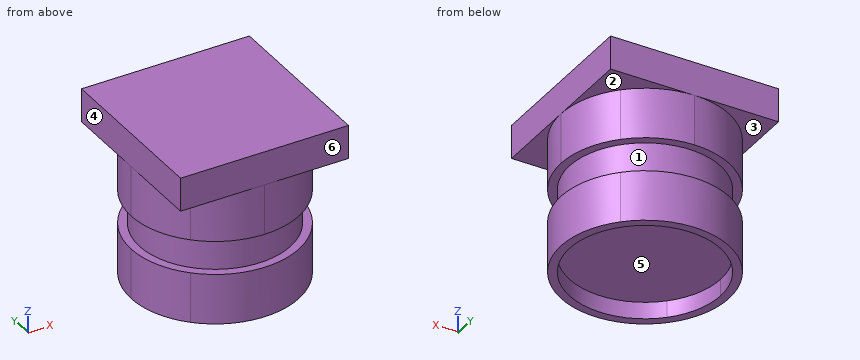
```python
from build123d import *

# Parameters (mm, degrees)
ESQUISSE1_W             = 10
ESQUISSE1_H             = 10
BOSS_EXTRU_1_DEPTH      = 2
BOSS_EXTRU_2_DEPTH      = 3
ESQUISSE3_R             = 4.5
BOSS_EXTRU_3_DEPTH      = 2
BOSS_EXTRU_5_DEPTH      = 3
ENL_V_START             = -1
ENL_V_MAT_EXTRU_1_DEPTH = 1


with BuildPart() as part:
    # Esquisse1 → Boss.-Extru.1 (new body)
    with BuildSketch(Plane.XY):
        with Locations((5, 1.73860374)):
            Rectangle(ESQUISSE1_W, ESQUISSE1_H)
    extrude(amount=BOSS_EXTRU_1_DEPTH)

    # Esquisse2 → Boss.-Extru.2 (add)
    with BuildSketch(Plane(origin=(0, 0, 0), x_dir=(-1, 0, 0), z_dir=(0, 0, -1))):
        with BuildLine():
            ThreePointArc((-5, 6.73860374), (-6.913417162, 6.358001403), (-8.535533906, 5.274137646))
            Line((-8.535533906, 5.274137646), (-1.464466094, -1.796930166))
            ThreePointArc((-1.464466094, -1.796930166), (-0.380602337, -0.174813421), (0, 1.73860374))
            ThreePointArc((0, 1.73860374), (-1.464466094, 5.274137646), (-5, 6.73860374))
        make_face()
        with BuildLine():
            Line((-1.464466094, -1.796930166), (-8.535533906, 5.274137646))
            ThreePointArc((-8.535533906, 5.274137646), (-9.619397663, 3.652020902), (-10, 1.73860374))
            ThreePointArc((-10, 1.73860374), (-8.535533906, -1.796930166), (-5, -3.26139626))
            ThreePointArc((-5, -3.26139626), (-3.086582838, -2.880793922), (-1.464466094, -1.796930166))
        make_face()
    extrude(amount=BOSS_EXTRU_2_DEPTH)

    # Esquisse3 → Boss.-Extru.3 (add)
    with BuildSketch(Plane(origin=(0, 0, -3), x_dir=(-1, 0, 0), z_dir=(0, 0, -1))):
        with Locations((-5, 1.73860374)):
            Circle(ESQUISSE3_R)
    extrude(amount=BOSS_EXTRU_3_DEPTH)

    # Esquisse4 → Boss.-Extru.5 (add)
    with BuildSketch(Plane(origin=(0, 0, -5), x_dir=(-1, 0, 0), z_dir=(0, 0, -1))):
        with BuildLine():
            ThreePointArc((0, 1.73860374), (-3.086582838, 6.358001403), (-8.535533906, 5.274137646))
            Line((-8.535533906, 5.274137646), (-8.181980515, 4.920584256))
            ThreePointArc((-8.181980515, 4.920584256), (-3.277924554, 5.896061637), (-0.5, 1.73860374))
            ThreePointArc((-0.5, 1.73860374), (-0.842542104, 0.016528295), (-1.818019485, -1.443376775))
            Line((-1.818019485, -1.443376775), (-1.464466094, -1.796930166))
            ThreePointArc((-1.464466094, -1.796930166), (-0.380602337, -0.174813421), (0, 1.73860374))
        make_face()
        with BuildLine():
            Line((-8.181980515, 4.920584256), (-8.535533906, 5.274137646))
            ThreePointArc((-8.535533906, 5.274137646), (-8.535533906, -1.796930166), (-1.464466094, -1.796930166))
            Line((-1.464466094, -1.796930166), (-1.818019485, -1.443376775))
            ThreePointArc((-1.818019485, -1.443376775), (-8.181980515, -1.443376775), (-8.181980515, 4.920584256))
        make_face()
        with BuildLine():
            ThreePointArc((-0.5, 1.73860374), (-3.277924554, 5.896061637), (-8.181980515, 4.920584256))
            Line((-8.181980515, 4.920584256), (-1.818019485, -1.443376775))
            ThreePointArc((-1.818019485, -1.443376775), (-0.842542104, 0.016528295), (-0.5, 1.73860374))
        make_face()
        with BuildLine():
            Line((-1.818019485, -1.443376775), (-8.181980515, 4.920584256))
            ThreePointArc((-8.181980515, 4.920584256), (-8.181980515, -1.443376775), (-1.818019485, -1.443376775))
        make_face()
    extrude(amount=BOSS_EXTRU_5_DEPTH)

    # Esquisse5 → Enlèv. mat.-Extru.1 (cut)
    with BuildSketch(Plane(origin=(0, 0, -8), x_dir=(-1, 0, 0), z_dir=(0, 0, -1)).offset(ENL_V_START)):
        with BuildLine():
            ThreePointArc((-0.5, 1.73860374), (-3.277924554, 5.896061637), (-8.181980515, 4.920584256))
            Line((-8.181980515, 4.920584256), (-1.818019485, -1.443376775))
            ThreePointArc((-1.818019485, -1.443376775), (-0.842542104, 0.016528295), (-0.5, 1.73860374))
        make_face()
        with BuildLine():
            Line((-1.818019485, -1.443376775), (-8.181980515, 4.920584256))
            ThreePointArc((-8.181980515, 4.920584256), (-8.181980515, -1.443376775), (-1.818019485, -1.443376775))
        make_face()
    extrude(amount=ENL_V_MAT_EXTRU_1_DEPTH, mode=Mode.SUBTRACT)


solid = part.part
```
CAD build for the part. Positions are in the model's coordinates, mm. Face numbers are marked on the shaded views. A direction names the side the tool comes from. Coordinates: 2 decimals unless noted, no trailing zeros. Order: outer loops, then holes, each group sorted by start corner. A loop starts at its lowest first (then second) coordinate and runs counter-clockwise, first axis right, second up. Notation, with made-up numbers: (-2, -8) - (17, -8) arc R25 cw to (17, 16) - close; hole circle Ø2 at (9, -27). An arc over 180 degrees is marked (long way). Use a Markdown table: item, result. Add a question column.
(1) Flat gauge pins, fed straight in: pin 1 (1 mm diameter, centred on x = 5, y = 0.5, fed in from -Z); pin 2 (3 mm diameter, centred on x = 3, z = -4.5, fed in from +Y). Where does each tip first touch, or does it go through?
(2) Which spindle directions (+Z, -Z, +X, -X, +Y, -Y) get a long thin tool onto all of the face, cutting with end or side? Do the marked faces 1, 2 and 3. Say none if no direction does.
(3) Drill centre lines: line 1 along Z through (x, y) = (1, 4.5); line 2 along Z through (x, y) = (7.5, 6.25); line 3 along Z through (x, y) = (1.5, 3.75). Where is each one in solid material? Low to high. Write a range as [from, to].
(4) Saw through at A-A (y = -1). Give the cut face in (x, z).
(5) Saw through at C-C (z = -1.5). Give the cut face in (x, y).
(6) Saw through at B-B (x = 3.25). Give the cut face in (y, z).
(7) Pull direction X, two halves, no side cores. Call the marked faces 4, 5 and 6: +X half, -X half, draft (parallel to the pull), parting line (faces both ways), or undercut.
Solved:
| question | item | result |
|---|---|---|
| 1 | pin 1 | stops at z = -7 |
| 1 | pin 2 | stops at y = 6.7 |
| 2 | face 1 | none |
| 2 | face 2 | -Z, +X, +Y |
| 2 | face 3 | -Z, -X, +Y |
| 3 | line 1 | z = [-8, -5], [-3, 2] |
| 3 | line 2 | z = [0, 2] |
| 3 | line 3 | z = [-7, 2] |
| 4 | outline | (0, 0) - (0.82, 0) - (0.82, -3) - (1.43, -3) - (1.43, -5) - (0.82, -5) - (0.82, -8) - (1.43, -8) - (1.43, -7) - (8.57, -7) - (8.57, -8) - (9.18, -8) - (9.18, -5) - (8.57, -5) - (8.57, -3) - (9.18, -3) - (9.18, 0) - (10, 0) - (10, 2) - (0, 2) - close |
| 5 | outline | circle Ø10 at (5, 1.74) |
| 6 | outline | (-3.26, 0) - (-2.95, 0) - (-2.95, -3) - (-2.41, -3) - (-2.41, -5) - (-2.95, -5) - (-2.95, -8) - (-2.41, -8) - (-2.41, -7) - (5.88, -7) - (5.88, -8) - (6.42, -8) - (6.42, -5) - (5.88, -5) - (5.88, -3) - (6.42, -3) - (6.42, 0) - (6.74, 0) - (6.74, 2) - (-3.26, 2) - close |
| 7 | face 4 | -X half |
| 7 | face 5 | undercut |
| 7 | face 6 | draft |
